from build123d import *

# Parameters (mm, degrees)
BOSS_EXTRUDE1_START = -5.08
SKETCH1_R           = 15.24
SKETCH1_R_2         = 1.5875
BOSS_EXTRUDE1_DEPTH = 2.8575
SKETCH2_R           = 3.81
SKETCH2_R_2         = 1.5875
BOSS_EXTRUDE2_DEPTH = 7.62
SKETCH3_R           = 1.190625


with BuildPart() as part:
    # Sketch1 → Boss-Extrude1 (new body)
    with BuildSketch(Plane.XY.offset(BOSS_EXTRUDE1_START)):
        Circle(SKETCH1_R)
        Circle(SKETCH1_R_2, mode=Mode.SUBTRACT)
    extrude(amount=BOSS_EXTRUDE1_DEPTH)

    # Sketch2 → Boss-Extrude2 (add)
    with BuildSketch(Plane.XY.offset(-2.2225)):
        with Locations(Location((0, 0, 0), (0, 0, 180))):
            Circle(SKETCH2_R)
        Circle(SKETCH2_R_2, mode=Mode.SUBTRACT)
    extrude(amount=BOSS_EXTRUDE2_DEPTH)

    # Sketch3 → Cut-Revolve1 (revolve, cut)
    with BuildSketch(Plane(origin=(0, 0, 0), x_dir=(1, 0, 0), z_dir=(0, 1, 0)), mode=Mode.PRIVATE) as cut_revolve1_sk:
        with Locations((3.81, -2.143125)):
            Circle(SKETCH3_R)
        with Locations((15.24, 3.65125)):
            Circle(SKETCH3_R)
    revolve(cut_revolve1_sk.sketch.rotate(Axis((0, 0, -2.2225), (0, 0, -1)), 180), axis=Axis((0, 0, -2.2225), (0, 0, -1)), mode=Mode.SUBTRACT)


solid = part.part
CAD build for the part. Positions are in the model's coordinates, mm. A direction names the side the tool comes from. Coordinates: 2 decimals unless noted, no trailing zeros. Loops run counter-clockwise (first coordinate to the right, second up) from the corner with the lowest first, then second, coordinate; pieces in that order, holes last. Notation, with made-up numbers: (-33, 75.5) - (-27, 75.5) arc R23 cw to (-27, 85.5) - close; hole circle Ø5 at (-18.75, 70). An arc over 180 degrees is marked (long way). Write item = value, one per line. Start each with the question number.
Q1. Cut at C-C, the plane z = 4.5. List the corners of the cut face in (x, y) (1 decimal), then the cut area to 3 significant figures.
Q2. Pull direction X, two halves, no side cores. Call faces 1 (the cylindrical face through (-0.34, -1.55, 0.09)), 2 (the cylindrical face through (0.496, -3.778, 4.351)), 3 (the flat face through (3, 0, -5.08)): pulls with the +X half, pulls with the -X half, needs draft (parallel to the pull), parting line crosses it, or undercut.
Q3. Cut at A-A, the plane y = 0. List the corners of the cut face in (x, z), then the cut area to 3 significant figures.
Q4. Drill centre lines: L1, parallel to Z at x = -8, y = -1.5; L2, parallel to X at y = 1, z = -3.25; L3, parallel to Y at x = 0, z = -2. Where is each one in solid material? Low to high.
Q5. Flat gauge pins, fed straight in: pin 1 Ø5 at (x, z) = (-8, 0.5) entering from -Y; pin 2 Ø10 at (x, y) = (3.5, 11.5) entering from +Z. Where does each tip first touch, or does it go through?
Q6. Which spindle directions (+Z, -Z, +X, -X, +Y, -Y) get a long thin tool onto all of the face, cutting with end or side? Do faces 4 (the flat face through (3, -3, -2.222)), 5 (the flat face through (0, 2, 5.398)). Say none if no direction does.
Q7. Cut at D-D, the plane z = -3.75. List the corners of the cut face in (x, y) (1 decimal), then the cut area to 3 significant figures.
Computed:
q1.outline = circle Ø7.6 at (0, 0); hole circle Ø3.2 at (0, 0)
q1.area = 37.7 mm²
q2.face_1 = undercut
q2.face_2 = parting line crosses it
q2.face_3 = needs draft
q3.outline = (-15.24, -5.08) - (-1.59, -5.08) - (-1.59, 5.4) - (-3.81, 5.4) - (-3.81, 3.33) arc R1.19 cw to (-3.81, 0.95) - (-3.81, -2.22) - (-15.24, -2.22) - (-15.24, -2.46) arc R1.19 cw to (-15.24, -4.84) - close; (1.59, -5.08) - (15.24, -5.08) - (15.24, -4.84) arc R1.19 cw to (15.24, -2.46) - (15.24, -2.22) - (3.81, -2.22) - (3.81, 0.95) arc R1.19 cw to (3.81, 3.33) - (3.81, 5.4) - (1.59, 5.4) - close
q3.area = 103 mm²
q4.L1 = -5.08 to -2.22
q4.L2 = -14.08 to -1.23, 1.23 to 14.08
q4.L3 = -3.81 to -1.59, 1.59 to 3.81
q5.pin_1 = through
q5.pin_2 = -2.22
q6.face_4 = +Z
q6.face_5 = +Z, +X, -X, +Y, -Y
q7.outline = circle Ø28.1 at (0, 0); hole circle Ø3.2 at (0, 0)
q7.area = 613 mm²
